```python
from build123d import *

# Parameters (mm, degrees)
F0_R      = 10
F1_DEPTH  = 5
F2_DEPTH  = 3
F3_R      = 3
F2_FACE_R = 7
F5_R      = 4.6788722556
F7_R      = 8
F7_R_2    = 4.6788722556
F8_DEPTH  = 2
F9_SIZE   = 1
F10_R     = 3.2686938503
F12_R     = 5.5
F14_SIZE  = 0.5
F15_R     = 2.3205955221
F16_DEPTH = 3
F17_R     = 2.3


with BuildPart() as f1:
    # F0 (on Top) → F1 (new body)
    with BuildSketch(Plane.XY):
        Circle(F0_R)
    extrude(amount=F1_DEPTH)

    # F2 (add): a face of the model
    f2_faces = [f1.faces().sort_by_distance(p)[0] for p in [
        (0, 0, 5),
    ]]
    extrude(f2_faces, amount=F2_DEPTH)

    # F3
    f3_edges = [f1.edges().sort_by_distance(p)[0] for p in [
        (-10, 0, 8),
    ]]
    fillet(f3_edges, radius=F3_R)

    # F2_face (on face) → F6 section 0
    with BuildSketch(Plane.XY.offset(8)):
        Circle(F2_FACE_R)
    # F5 (on offset) → F6 section 1
    with BuildSketch(Plane.XY.offset(28)):
        Circle(F5_R)
    loft()

    # F7 (on face) → F8 (join)
    with BuildSketch(Plane.XY.offset(28)):
        Circle(F7_R)
        Circle(F7_R_2, mode=Mode.SUBTRACT)
        Circle(F7_R_2)
    extrude(amount=F8_DEPTH)

    # F9
    f9_edges = [f1.edges().sort_by_distance(p)[0] for p in [
        (-8, 0, 30),
    ]]
    chamfer(f9_edges, length=F9_SIZE)

    # F10 (on face) → F13 section 0
    with BuildSketch(Plane.XY.offset(30)):
        Circle(F10_R)
    # F12 (on offset) → F13 section 1
    with BuildSketch(Plane.XY.offset(40)):
        Circle(F12_R)
    loft()

    # F14
    f14_edges = [f1.edges().sort_by_distance(p)[0] for p in [
        (-5.5, 0, 40),
    ]]
    chamfer(f14_edges, length=F14_SIZE)

    # F15 (on face) → F16 (join)
    with BuildSketch(Plane.XY.offset(40)):
        Circle(F15_R)
    extrude(amount=F16_DEPTH)

    # F17
    f17_edges = [f1.edges().sort_by_distance(p)[0] for p in [
        (-2.320596, 0, 43),
    ]]
    fillet(f17_edges, radius=F17_R)


solid = f1.part
```
Can you work these out from the model? Positions are in its coordinate system, mm. A direction names the side the tool comes from. Give positions to 0.01 mm unless a question says otherwise; leave off trailing zeros. Loops run counter-clockwise (first coordinate to the right, second up) from the corner with the lowest first, then second, coordinate; pieces in that order, holes last. Notation, with made-up numbers: M 79.25,3.25 L 130.25,3.25 A19 cw 130.25,23.25 Z; hole C 10.5,-30.5 d9. An arc over 180 degrees is marked long. One line per question, with ' | ' between items. Start each with the question number.
Q1. For faces 1 (the cylindrical face through (-1.73, -7.81, 28.49)), 2 (the conical face through (-0.758, 5.774, 18.14)), 3 (the cylindrical face through (-2.17, -9.76, 2.46)), which set-ups out of +Z, -Z, +X, -X, +Y, -Y let a thin tool reach every point of the face, with its end or its side?
Q2. If I drill on line 1 (X direction, y = 8.75, z = 4); line 2 (Y direction, x = 1, z = 22); line 3 (Y direction, x = 7, z = 3), over which ranges is the centre line in solid material (lowest first)? Write a range as from..to.
Q3. For pin 1 Ø3 at (x, y) = (6.5, -4) entering from -Z; pin 2 Ø1.5 at (x, z) = (6, 27.5) entering from +Y; pin 3 Ø4 at (x, y) = (-3.5, -3) entering from +Z; pin 4 Ø10 at (x, z) = (3.5, 12) entering from -Y, each with a flat end and sliding along its axis, tell me the tip position at first contact or that it passes through.
Q4. If we section it at A-A (z = 21.5): Please give me the cut outline in (x, y), plus the area to 3 significant figures.
Q5. If we mould it in two halves opening along Z, with no side actions, what happens to faces 4 (the cylindrical face through (2.213, 0.697, 40.345)), 5 (the flat face through (2.2, 1.2, 40)), 6 (the flat face through (0, 0, 0)), 7 (the flat face through (3, 2, 30))? For each: +Z half, -Z half, draft (parallel to the pull), parting line (faces both ways), or undercut.
Q6. If we section it at B-B (z = 30.5): Please give me the cut outline in (x, y), plus the area to 3 significant figures.
Computed:
1) face 1: +Z | face 2: none | face 3: +Z, -Z
2) line 1: x = -4.84..4.84 | line 2: y = -5.28..5.28 | line 3: y = -7.14..7.14
3) pin 1: stops at z = 0 | pin 2: stops at y = 5.86 | pin 3: stops at z = 40 | pin 4: stops at y = -8.8
4) outline: C 0,0 d10.87 | area: 92.7 mm²
5) face 4: draft | face 5: +Z half | face 6: -Z half | face 7: undercut
6) outline: C 0,0 d6.76 | area: 35.9 mm²
